Check sheet for the modelled part. Datum: model origin and axes. Units: mm. Face numbers are marked on the shaded views. A direction names the side the tool comes from. Give positions to 0.01 mm unless a question says otherwise; leave off trailing zeros. Write each loop counter-clockwise with the first axis right and the second up, starting at its lowest first coordinate (ties: lowest second). Pieces come first, ordered by that corner, then holes.
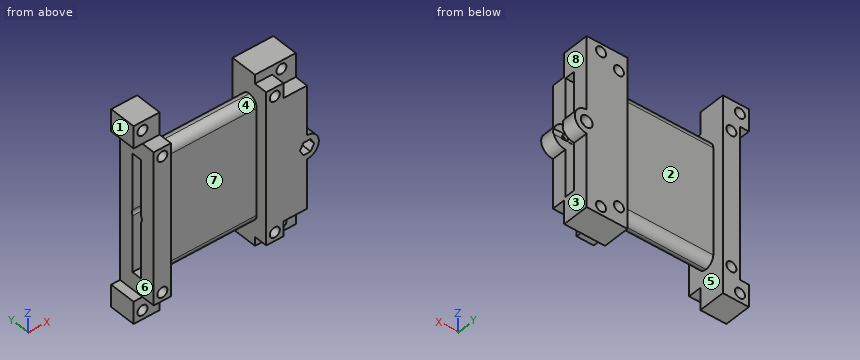
from build123d import *

# Parameters (mm, degrees)
SKETCH1_W              = 42
SKETCH1_H              = 5.9
SKETCH1_W_2            = 39.9
SKETCH1_H_2            = 3.5
BOSS_EXTRUDE1_DEPTH    = 32.25
FILLET2_R              = 3
SKETCH2_W              = 51.5
SKETCH2_H              = 13.6
SKETCH2_W_2            = 39.9
SKETCH2_H_2            = 3.5
BOSS_EXTRUDE2_DEPTH    = 5.8
SKETCH3_W              = 51.5
SKETCH3_H              = 13.6
SKETCH3_W_2            = 39.9
SKETCH3_H_2            = 3.5
BOSS_EXTRUDE3_DEPTH    = 5.8
SKETCH4_R              = 1.7
CUT_EXTRUDE1_DEPTH     = 62.792596644
SKETCH8_W              = 8.8
SKETCH8_H              = 7.5
BOSS_EXTRUDE4_DEPTH    = 13.6
CUT_EXTRUDE4_DEPTH     = 4
SKETCH15_W             = 39.9
SKETCH15_H             = 3.5
CUT_EXTRUDE5_DEPTH     = 79.468767672
SKETCH17_R             = 2
CUT_EXTRUDE6_DEPTH     = 79.468767672
M3_CLEARANCE_HOLE1_D   = 3.4
CUT_EXTRUDE8_START     = -13.6
CUT_EXTRUDE8_OUTLINE_W = 8.8
CUT_EXTRUDE8_OUTLINE_H = 7.5
CUT_EXTRUDE8_OUTLINE_R = 1.7
CUT_EXTRUDE8_DEPTH     = 4.55


# Read off the part's stored shape, not the designer's step: Cut-Extrude8
with BuildPart() as part:
    # Sketch1 → Boss-Extrude1 (new body)
    with BuildSketch(Plane(origin=(0, 0, 0), x_dir=(0, 0, -1), z_dir=(1, 0, 0))):
        with Locations((21, 2.95)):
            Rectangle(SKETCH1_W, SKETCH1_H)
        with Locations((21, 2.95)):
            Rectangle(SKETCH1_W_2, SKETCH1_H_2, mode=Mode.SUBTRACT)
    extrude(amount=BOSS_EXTRUDE1_DEPTH)

    # Fillet2
    # the kernel refuses this fillet: 3 mm, written as the material it takes off along each edge
    with BuildSketch(Plane(origin=(-7.5, 0, -42), x_dir=(0, 0, 1), z_dir=(1, 0, 0)), Plane(origin=(-7.5, 5.9, 0), x_dir=(0, 0, -1), z_dir=(1, 0, 0)), Plane(origin=(-7.5, 5.9, -42), x_dir=(0, -1, 0), z_dir=(1, 0, 0))) as fillet2_piece_1:
        with BuildLine():
            CenterArc((FILLET2_R, -FILLET2_R), FILLET2_R, 90, 90)
            Line((0, -FILLET2_R), (0, 0))
            Line((0, 0), (FILLET2_R, 0))
        make_face()
    extrude(amount=47.25, mode=Mode.SUBTRACT)
    with BuildSketch(Plane(origin=(-7.5, 0, 0), x_dir=(0, 0, -1), z_dir=(1, 0, 0))) as fillet2_piece_2:
        with BuildLine():
            CenterArc((FILLET2_R, FILLET2_R), FILLET2_R, 180, 90)
            Line((0, FILLET2_R), (0, 0))
            Line((0, 0), (FILLET2_R, 0))
        make_face()
    extrude(amount=47.25, mode=Mode.SUBTRACT)

    # Sketch2 → Boss-Extrude2 (add)
    with BuildSketch(Plane(origin=(32.25, 0, 0), x_dir=(0, 0, -1), z_dir=(1, 0, 0))):
        with Locations((21, 2.95)):
            Rectangle(SKETCH2_W, SKETCH2_H)
        with Locations((21, 2.95)):
            Rectangle(SKETCH2_W_2, SKETCH2_H_2, mode=Mode.SUBTRACT)
    extrude(amount=BOSS_EXTRUDE2_DEPTH)

    # Sketch3 → Boss-Extrude3 (add)
    with BuildSketch(Plane.ZY):
        with Locations((-21, 2.95)):
            Rectangle(SKETCH3_W, SKETCH3_H)
        with Locations((-21, 2.95)):
            Rectangle(SKETCH3_W_2, SKETCH3_H_2, mode=Mode.SUBTRACT)
    extrude(amount=BOSS_EXTRUDE3_DEPTH)

    # Sketch4 → Cut-Extrude1 (cut, through all)
    with BuildSketch(Plane(origin=(0, 9.75, 0), x_dir=(1, 0, 0), z_dir=(0, 1, 0))):
        with Locations(Location((-2.9, 43.85, 0), (0, 0, 270))):
            Circle(SKETCH4_R)
        with Locations(Location((35.15, 43.85, 0), (0, 0, 270))):
            Circle(SKETCH4_R)
        with Locations(Location((-2.9, -1.85, 0), (0, 0, 270))):
            Circle(SKETCH4_R)
        with Locations(Location((35.15, -1.85, 0), (0, 0, 270))):
            Circle(SKETCH4_R)
    extrude(amount=-CUT_EXTRUDE1_DEPTH, mode=Mode.SUBTRACT)

    # Sketch8 → Boss-Extrude4 (add)
    with BuildSketch(Plane(origin=(0, 9.75, 0), x_dir=(1, 0, 0), z_dir=(0, 1, 0))):
        with Locations((-4.4, 50.5)):
            Rectangle(SKETCH8_W, SKETCH8_H)
        with Locations((-4.4, -8.5)):
            Rectangle(SKETCH8_W, SKETCH8_H)
        with BuildLine():
            Line((46.05, 25), (46.05, 49.75))
            Line((46.05, 49.75), (32.25, 49.75))
            Line((32.25, 49.75), (32.25, 46.75))
            Line((32.25, 46.75), (38.05, 46.75))
            Line((38.05, 46.75), (38.05, -4.75))
            Line((38.05, -4.75), (32.25, -4.75))
            Line((32.25, -4.75), (32.25, -7.75))
            Line((32.25, -7.75), (46.05, -7.75))
            Line((46.05, -7.75), (46.05, 17))
            ThreePointArc((46.05, 17), (50.05, 21), (46.05, 25))
        make_face()
    extrude(amount=-BOSS_EXTRUDE4_DEPTH)

    # Sketch13 → CSK for M2 Flat Head Machine Screw1 (revolve, cut)
    with BuildSketch(Plane(origin=(46.05, 9.75, -21), x_dir=(0, 0, 1), z_dir=(1, 0, 0))):
        Polygon((0, 0), (0, 13.6), (1, 13.6), (1, 3.75), (2, 2.75), (2, 0), align=None)
    revolve(axis=Axis((46.05, 16.1, -21), (0, -1, 0)), mode=Mode.SUBTRACT)

    # Sketch14 → Cut-Extrude4 (cut)
    with BuildSketch(Plane.XZ.offset(3.85)):
        Polygon((43.625128869, -21), (44.837564435, -23.1), (47.262435565, -23.1), (48.474871131, -21), (47.262435565, -18.9), (44.837564435, -18.9), align=None)
    extrude(amount=-CUT_EXTRUDE4_DEPTH, mode=Mode.SUBTRACT)

    # Sketch15 → Cut-Extrude5 (cut, through all)
    with BuildSketch(Plane.ZY.offset(5.8)):
        with Locations((-21, 2.95)):
            Rectangle(SKETCH15_W, SKETCH15_H)
    extrude(amount=-CUT_EXTRUDE5_DEPTH, mode=Mode.SUBTRACT)

    # Sketch17 → Cut-Extrude6 (cut, through all)
    with BuildSketch(Plane.ZY.offset(5.8)):
        with Locations((-21, 2.95)):
            Circle(SKETCH17_R)
    extrude(amount=-CUT_EXTRUDE6_DEPTH, mode=Mode.SUBTRACT)

    # M3 Clearance Hole1 (through all)
    with Locations(Plane(origin=(-5.8, 9.75, -51.25), x_dir=(0, 0, 1), z_dir=(0, 1, 0))):
        with Locations((0, 0), (4.25, 47), (56.25, 47), (60.5, 0)):
            Hole(M3_CLEARANCE_HOLE1_D / 2)

    # Cut-Extrude8 outline → Cut-Extrude8 (cut)
    # profile 1 of 4: a face of its own
    with BuildSketch(Plane(origin=(0, 9.75, 0), x_dir=(1, 0, 0), z_dir=(0, 1, 0)).offset(CUT_EXTRUDE8_START)):
        with Locations((-4.4, 50.5)):
            Rectangle(CUT_EXTRUDE8_OUTLINE_W, CUT_EXTRUDE8_OUTLINE_H)
        with Locations((-5.8, 51.25)):
            Circle(CUT_EXTRUDE8_OUTLINE_R, mode=Mode.SUBTRACT)
    # profile 2 of 4: a face of its own
    with BuildSketch(Plane(origin=(0, 9.75, 0), x_dir=(1, 0, 0), z_dir=(0, 1, 0)).offset(CUT_EXTRUDE8_START)):
        with Locations((-4.4, -8.5)):
            Rectangle(CUT_EXTRUDE8_OUTLINE_W, CUT_EXTRUDE8_OUTLINE_H)
        with Locations((-5.8, -9.25)):
            Circle(CUT_EXTRUDE8_OUTLINE_R, mode=Mode.SUBTRACT)
    # profile 3 of 4: a face of its own
    with BuildSketch(Plane(origin=(0, 9.75, 0), x_dir=(1, 0, 0), z_dir=(0, 1, 0)).offset(CUT_EXTRUDE8_START)):
        Polygon((32.25, 49.75), (32.25, 46.75), (38.05, 46.75), (38.05, 41.7), (46.05, 41.7), (46.05, 49.75), align=None)
        with Locations((41.2, 47)):
            Circle(CUT_EXTRUDE8_OUTLINE_R, mode=Mode.SUBTRACT)
    # profile 4 of 4: a face of its own
    with BuildSketch(Plane(origin=(0, 9.75, 0), x_dir=(1, 0, 0), z_dir=(0, 1, 0)).offset(CUT_EXTRUDE8_START)):
        Polygon((38.05, -4.75), (32.25, -4.75), (32.25, -7.75), (46.05, -7.75), (46.05, 0.3), (38.05, 0.3), align=None)
        with Locations((41.2, -5)):
            Circle(CUT_EXTRUDE8_OUTLINE_R, mode=Mode.SUBTRACT)
    extrude(amount=CUT_EXTRUDE8_DEPTH, mode=Mode.SUBTRACT)


solid = part.part
1) Sectioned sample at A-A on y = -1.5. Record the boundary of the cut face in (x, z), then the cut area to 3 significant figures.
2) Sectioned sample at C-C on x = 41.2. Record the boundary of the cut face in (y, z).
3) Sectioned sample at D-D on z = -33. Record the boundary of the cut face in (x, y).
4) Access from +Z, -Z, +X, -X, +Y, -Y to the whole of each face (thin tool, end or side, straight path). Record for the marked faces 5, 6, 7 and 8.
5) Draft check along X on the marked faces 1, 2, 3 and 4. Enter one of: +X half, -X half, draft (parallel to the pull), parting line (faces both ways), or undercut.
6) Scan lines: L1, parallel to X at y = 5.5, z = -47; L2, parallel to X at y = 3.75, z = 1.85; L3, parallel to X at y = 5.75, z = -41.5. Record each from-to range of solid material in increasing order.
7) Gauge pin test, flat ends, axial feed: pin 1 (4 mm diameter, centred on y = 4, z = -7, fed in from -X); pin 2 (4 mm diameter, centred on y = 1, z = -13.5, fed in from +X); pin 3 (1.8 mm diameter, centred on x = 46.05, z = -21, fed in from +Y); pin 4 (2 mm diameter, centred on x = -5.5, z = -49, fed in from -Y). Record the tip position at first contact, or that the pin passes through.
8) Sectioned sample at B-B on z = -43.85. Record the boundary of the cut face in (x, y).
Answers below:
1. outline: (-5.8, -46.75) - (0, -46.75) - (0, 4.75) - (-5.8, 4.75) - close; (32.25, -46.75) - (38.05, -46.75) - (38.05, -41.7) - (46.05, -41.7) - (46.05, -25) arc R4 ccw to (46.05, -17) - (46.05, -0.3) - (38.05, -0.3) - (38.05, 4.75) - (32.25, 4.75) - close; hole circle Ø3.4 at (-2.9, -43.85); hole circle Ø3.4 at (-2.9, 1.85); hole circle Ø3.4 at (35.15, -43.85); hole circle Ø3.4 at (35.15, 1.85); hole (43.63, -21) - (44.84, -23.1) - (47.26, -23.1) - (48.47, -21) - (47.26, -18.9) - (44.84, -18.9) - close
1. area: 902 mm2
2. outline: (-3.85, -41.7) - (0.7, -41.7) - (0.7, -45.3) - (9.75, -45.3) - (9.75, 3.3) - (0.7, 3.3) - (0.7, -0.3) - (-3.85, -0.3) - close; (0.7, -49.75) - (9.75, -49.75) - (9.75, -48.7) - (0.7, -48.7) - close; (0.7, 6.7) - (9.75, 6.7) - (9.75, 7.75) - (0.7, 7.75) - close; hole (1.2, -40.95) - (4.7, -40.95) - (4.7, -21.97) arc R2 ccw to (4.7, -20.03) - (4.7, -1.05) - (1.2, -1.05) - (1.2, -20.03) arc R2 ccw to (1.2, -21.97) - close
3. outline: (-5.8, -3.85) - (0, -3.85) - (0, 0) - (32.25, 0) - (32.25, -3.85) - (46.05, -3.85) - (46.05, 1.2) - (-5.8, 1.2) - close; (-5.8, 4.7) - (46.05, 4.7) - (46.05, 9.75) - (32.25, 9.75) - (32.25, 5.9) - (0, 5.9) - (0, 9.75) - (-5.8, 9.75) - close
4. face 5: none
4. face 6: -X, +Y, -Y
4. face 7: +Z, -Z, -Y
4. face 8: +Z, +X, +Y, -Y
5. face 1: -X half
5. face 2: undercut
5. face 3: +X half
5. face 4: undercut
6. L1: x = -8.8 to 0, 32.25 to 39.5, 42.9 to 46.05
6. L2: x = -5.8 to -4.6, -1.2 to 0, 32.25 to 33.45, 36.85 to 46.05
6. L3: x = -5.8 to 0, 32.25 to 46.05
7. pin 1: stops at x = -5.8
7. pin 2: stops at x = 46.05
7. pin 3: passes through
7. pin 4: stops at y = 0.7
8. outline: (-5.8, -3.85) - (-4.6, -3.85) - (-4.6, 9.75) - (-5.8, 9.75) - close; (-1.2, -3.85) - (0, -3.85) - (0, 9.75) - (-1.2, 9.75) - close; (32.25, -3.85) - (33.45, -3.85) - (33.45, 9.75) - (32.25, 9.75) - close; (36.85, -3.85) - (38.05, -3.85) - (38.05, 0.7) - (46.05, 0.7) - (46.05, 9.75) - (36.85, 9.75) - close
